Geometry check sheet. Reference: the model listing, model coordinates, mm. Give positions to 0.01 mm unless a question says otherwise; leave off trailing zeros. Write each loop counter-clockwise with the first axis right and the second up, starting at its lowest first coordinate (ties: lowest second). Pieces come first, ordered by that corner, then holes. Notation, with made-up numbers: (86.25, 73) - (94.25, 73) arc R21 cw to (94.25, 104) - close; hole circle Ø10 at (36, -39.75). An arc over 180 degrees is marked (long way). Write item = value, one per line. Start each with the question number.
(1) Section check A-A, the plane y = 42. Enter the section's corners in (x, z).
(2) Section check B-B, the plane z = 2.05. Give the number of separate pieces and of enclosed holes in the cut face, plus the area to 3 significant figures.
(3) Thickness scan on L1, parallel to X at y = 27.5, z = 1.05; L2, parallel to Y at x = -9.5, z = 1.05; L3, parallel to Y at x = -6.5, z = 3.15. Record the ranges inside material, lowest first.
(4) Section check D-D, the plane y = 9. Enter the section's corners in (x, z), plus the area to 3 significant figures.
(5) Depth check by flat-ended pin: pin 1 Ø1 at (y, z) = (-19.5, 3) entering from -X. Enter the tip coordinate at first touch or a pass-through.
(6) Draft check along Y on faces 1 (the flat face through (-1, 1, 0)), 2 (the cylindrical face through (-55.55, -42.594, 2.465)), 3 (the cylindrical face through (52.85, 31.39, 2.46)). Enter one of: pulls with the +Y half, pulls with the -Y half, needs draft (parallel to the pull), parting line crosses it, or undercut.
(7) Section check C-C, the plane x = -56. Enter the section's corners in (y, z).
```python
from build123d import *

# Parameters (mm, degrees)
SKETCH1_R           = 70
SKETCH1_R_2         = 1.65
SKETCH1_R_3         = 4
SKETCH1_R_4         = 1.5
BOSS_EXTRUDE1_DEPTH = 5
SKETCH2_R           = 2
CUT_EXTRUDE1_DEPTH  = 100.121138008


with BuildPart() as part:
    # Sketch1 → Boss-Extrude1 (new body)
    with BuildSketch(Plane.XY):
        Circle(SKETCH1_R)
        with Locations((0, 60)):
            Circle(SKETCH1_R_2, mode=Mode.SUBTRACT)
        with Locations((51.961524227, 30)):
            Circle(SKETCH1_R_2, mode=Mode.SUBTRACT)
        with Locations((51.961524227, -30)):
            Circle(SKETCH1_R_2, mode=Mode.SUBTRACT)
        with Locations((0, -60)):
            Circle(SKETCH1_R_2, mode=Mode.SUBTRACT)
        with Locations((-51.961524227, -30)):
            Circle(SKETCH1_R_2, mode=Mode.SUBTRACT)
        with Locations((-51.961524227, 30)):
            Circle(SKETCH1_R_2, mode=Mode.SUBTRACT)
        with Locations((0, 29)):
            Circle(SKETCH1_R_3, mode=Mode.SUBTRACT)
        with Locations((7.794228634, 24.5)):
            Circle(SKETCH1_R_3, mode=Mode.SUBTRACT)
        with Locations((7.794228634, 15.5)):
            Circle(SKETCH1_R_3, mode=Mode.SUBTRACT)
        with Locations((0, 11)):
            Circle(SKETCH1_R_3, mode=Mode.SUBTRACT)
        with Locations((-7.794228634, 15.5)):
            Circle(SKETCH1_R_3, mode=Mode.SUBTRACT)
        with Locations((-7.794228634, 24.5)):
            Circle(SKETCH1_R_3, mode=Mode.SUBTRACT)
        with Locations((0, 20)):
            Circle(SKETCH1_R_4, mode=Mode.SUBTRACT)
        with Locations(Location((7.794228634, -15.5, 0), (0, 0, 180))):
            Circle(SKETCH1_R_3, mode=Mode.SUBTRACT)
        with Locations(Location((0, -11, 0), (0, 0, 180))):
            Circle(SKETCH1_R_3, mode=Mode.SUBTRACT)
        with Locations(Location((-7.794228634, -15.5, 0), (0, 0, 180))):
            Circle(SKETCH1_R_3, mode=Mode.SUBTRACT)
        with Locations(Location((0, -20, 0), (0, 0, 180))):
            Circle(SKETCH1_R_4, mode=Mode.SUBTRACT)
        with Locations(Location((-7.794228634, -24.5, 0), (0, 0, 180))):
            Circle(SKETCH1_R_3, mode=Mode.SUBTRACT)
        with Locations(Location((0, -29, 0), (0, 0, 180))):
            Circle(SKETCH1_R_3, mode=Mode.SUBTRACT)
        with Locations(Location((7.794228634, -24.5, 0), (0, 0, 180))):
            Circle(SKETCH1_R_3, mode=Mode.SUBTRACT)
    extrude(amount=BOSS_EXTRUDE1_DEPTH)

    # Sketch2 → Cut-Extrude1 (cut, through all)
    with BuildSketch(Plane.XY.offset(5)):
        with Locations((0, 42)):
            Circle(SKETCH2_R)
        with Locations((0, -42)):
            Circle(SKETCH2_R)
        with Locations((18, 0)):
            Circle(SKETCH2_R)
        with Locations((-18, 0)):
            Circle(SKETCH2_R)
    extrude(amount=-CUT_EXTRUDE1_DEPTH, mode=Mode.SUBTRACT)


solid = part.part
```
Model answer:
q1.outline = (-56, 0) - (-2, 0) - (-2, 5) - (-56, 5) - close; (2, 0) - (56, 0) - (56, 5) - (2, 5) - close
q2.separate_pieces = 1
q2.enclosed_holes = 24
q2.area = 14,700 mm²
q3.L1 = -64.37 to -10.44, -5.15 to -3.71, 3.71 to 5.15, 10.44 to 64.37
q3.L2 = -69.35 to -28.12, -20.88 to -19.12, -11.88 to 11.88, 19.12 to 20.88, 28.12 to 69.35
q3.L3 = -69.7 to -28.28, -20.72 to -19.28, -11.72 to 11.72, 19.28 to 20.72, 28.28 to 69.7
q4.outline = (-69.42, 0) - (-3.46, 0) - (-3.46, 5) - (-69.42, 5) - close; (3.46, 0) - (69.42, 0) - (69.42, 5) - (3.46, 5) - close
q4.area = 660 mm²
q5.pin_1 = -67.37
q6.face_1 = needs draft
q6.face_2 = parting line crosses it
q6.face_3 = undercut
q7.outline = (-42, 0) - (42, 0) - (42, 5) - (-42, 5) - close
